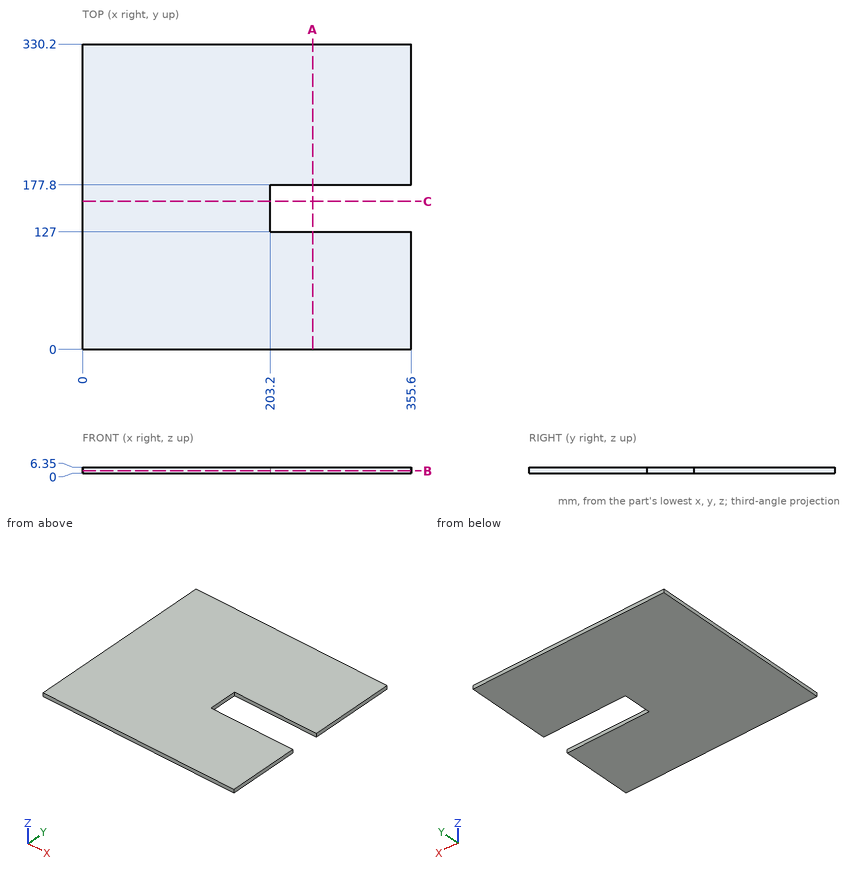
Verification items for this drawing (mm, ordinates from the low corner). Coordinates: 2 decimals unless noted, no trailing zeros. Loops run counter-clockwise (first coordinate to the right, second up) from the corner with the lowest first, then second, coordinate; pieces in that order, holes last.
Item 1: Thickness scan on line 1 (Y direction, x = 329, z = 5.75); line 2 (X direction, y = 131, z = 3.25). Record the ranges inside material, lowest first.
Item 2: Sectioned sample at C-C, the plane y = 160. Record the boundary of the cut face in (x, z).
Item 3: Sectioned sample at A-A, the plane x = 249. Record the boundary of the cut face in (y, z), then the cut area to 3 significant figures.
Item 4: Sectioned sample at B-B, the plane z = 2.5. Record the boundary of the cut face in (x, y).
Check result:
1. line 1: y = 0 to 127, 177.8 to 330.2
1. line 2: x = 0 to 203.2
2. outline: (0, 0) - (203.2, 0) - (203.2, 6.35) - (0, 6.35) - close
3. outline: (0, 0) - (127, 0) - (127, 6.35) - (0, 6.35) - close; (177.8, 0) - (330.2, 0) - (330.2, 6.35) - (177.8, 6.35) - close
3. area: 1,770 mm2
4. outline: (0, 0) - (355.6, 0) - (355.6, 127) - (203.2, 127) - (203.2, 177.8) - (355.6, 177.8) - (355.6, 330.2) - (0, 330.2) - close
